```python
from build123d import *

# Parameters (mm, degrees)
SKETCH_1_R          = 25
SKETCH_1_R_2        = 20
EXTRUDE_3_DEPTH     = 25
SKETCH_12_R         = 1.5
CUT_EXTRUDE_3_DEPTH = 15
SKETCH_13_R         = 30
EXTRUDE_5_DEPTH     = 5


with BuildPart() as part:
    # 草图1 → 凸台-拉伸3 (new body)
    with BuildSketch(Plane.XY):
        with Locations((-41.161572615, 8.306984042)):
            Circle(SKETCH_1_R)
        with Locations((-41.161572615, 8.306984042)):
            Circle(SKETCH_1_R_2, mode=Mode.SUBTRACT)
    extrude(amount=EXTRUDE_3_DEPTH)

    # 草图12 → 切除-拉伸3 (cut)
    with BuildSketch(Plane(origin=(0, 0, 0), x_dir=(-1, 0, 0), z_dir=(0, 0, -1))):
        with Locations((41.161572615, 30.806984042)):
            Circle(SKETCH_12_R)
        with Locations((63.661572615, 8.306984042)):
            Circle(SKETCH_12_R)
        with Locations((41.161572615, -14.193015958)):
            Circle(SKETCH_12_R)
        with Locations((18.661572615, 8.306984042)):
            Circle(SKETCH_12_R)
    extrude(amount=-CUT_EXTRUDE_3_DEPTH, mode=Mode.SUBTRACT)

    # 草图13 → 凸台-拉伸5 (add)
    with BuildSketch(Plane.XY.offset(25)):
        with Locations((-41.161572615, 8.306984042)):
            Circle(SKETCH_13_R)
    extrude(amount=EXTRUDE_5_DEPTH)


solid = part.part
```
The model under review builds one solid part; all positions refer to its coordinate system, in mm. A direction names the side the tool comes from. Coordinates: 2 decimals unless noted, no trailing zeros. Order: outer loops, then holes, each group sorted by start corner. A loop starts at its lowest first (then second) coordinate and runs counter-clockwise, first axis right, second up. Notation, with made-up numbers: M 62,43 L 93,43 A16 ccw 93,49 Z; hole C 88,-4 d5. An arc over 180 degrees is marked long. One line per question, with ' | ' between items.
(1) Insertion check: pin 1 (5 mm diameter, centred on x = -64.5, z = 3.5, fed in from +Y); pin 2 (8 mm diameter, centred on x = -45.5, z = 24, fed in from +Y); pin 3 (20 mm diameter, centred on x = -47, y = 15, fed in from -Z). Each pin has a flat end and moves straight along its axis. Give the tip position at first contact, or say it passes through.
Geometry results:
pin 1: stops at y = 22.12 | pin 2: stops at y = 38.3 | pin 3: stops at z = 25
(2) For probe 1 along Y at (x, z) = (-42.5, 6); probe 2 along Z at (x, y) = (-18, -10.5); probe 3 along X at (y, z) = (10, 23.75), list the stretches that pass through material, from the lowest coordinate up. Write a range as from..to.
Geometry results:
probe 1: y = -16.66..-14.87, -13.52..-11.65, 28.26..30.13, 31.48..33.27 | probe 2: z = 25..30 | probe 3: x = -66.1..-61.09, -21.23..-16.22
(3) Add section C-C, the plane z = 11.5. Write out the cut boundary in (x, y), then the cut area to 3 significant figures.
Geometry results:
outline: C -41.16,8.31 d50; hole C -63.66,8.31 d3; hole C -41.16,8.31 d40; hole C -41.16,-14.19 d3; hole C -41.16,30.81 d3; hole C -18.66,8.31 d3 | area: 679 mm²
(4) The part is to be moulded in two halves that separate along Y. For faces 1 (the face through (-42, 9, 30)), 2 (the face through (-59.59, 25.2, 12.32)), 3 (the face through (-62.471, 7.394, 7.395)), 4 (the face through (-61.142, 9.186, 12.325)), say which applies: +Y half, -Y half, draft (parallel to the pull), parting line (faces both ways), or undercut.
Geometry results:
face 1: draft | face 2: parting line | face 3: undercut | face 4: undercut
(5) Add section B-B, the plane y = -9.5. Write out the cut boundary in (x, z), then the cut area to 3 significant figures.
Geometry results:
outline: M -65.31,25 L -58.71,25 L -58.71,0 L -50.27,0 L -50.27,25 L -32.06,25 L -32.06,0 L -23.61,0 L -23.61,25 L -17.02,25 L -17.02,30 L -65.31,30 Z | area: 664 mm²
(6) Add section D-D, the plane z = 20.5. Write out the cut boundary in (x, y).
Geometry results:
outline: C -41.16,8.31 d50; hole C -41.16,8.31 d40
(7) Machinability: for faces 5 (the face through (-49, 27, 0)), 6 (the face through (-19, 8, 15)), which of the approach directions +Z, -Z, +X, -X, +Y, -Y give a long, thin tool a straight path to every point of the face, cutting with its end or side? Answer none if there is none.
Geometry results:
face 5: -Z, +X, -X, +Y, -Y | face 6: -Z
(8) Add section A-A, the plane x = -24.5. Write out the cut boundary in (y, z).
Geometry results:
outline: M -16.64,25 L -10.33,25 L -10.33,0 L -2.76,0 L -2.76,25 L 19.37,25 L 19.37,0 L 26.95,0 L 26.95,25 L 33.25,25 L 33.25,30 L -16.64,30 Z
